```python
from build123d import *

# Parameters (mm, degrees)
F0_W      = 1520
F0_H      = 750
F1_DEPTH  = 25
F2_W      = 1470
F2_H      = 25
F3_DEPTH  = 25
F5_DEPTH  = 65
F7_W      = 25
F7_H      = 25
F8_DEPTH  = 675
F10_DEPTH = 65
F12_W     = 25
F12_H     = 25
F13_DEPTH = 675
F15_W     = 25
F15_H     = 25
F16_DEPTH = 675
F18_W     = 25
F18_H     = 25
F19_DEPTH = 650
F21_W     = 25
F21_H     = 25
F22_DEPTH = 650
F24_DEPTH = 10
F26_DEPTH = 10
F29_DEPTH = 10
F31_DEPTH = 10


with BuildPart() as f1:
    # F0 (on Top) → F1 (new body)
    with BuildSketch(Plane.XY):
        with Locations((-760, 375)):
            Rectangle(F0_W, F0_H)
    extrude(amount=F1_DEPTH)

    # F2 (on face) → F3 (join)
    with BuildSketch(Plane(origin=(0, 0, 0), x_dir=(1, 0, 0), z_dir=(0, 0, -1))):
        with Locations((-760, -37.5)):
            Rectangle(F2_W, F2_H)
        with Locations((-760, -712.5)):
            Rectangle(F2_W, F2_H)
    extrude(amount=F3_DEPTH)

    # F4 (on face) → F5 (join)
    with BuildSketch(Plane(origin=(0, 0, 0), x_dir=(1, 0, 0), z_dir=(0, 0, -1))):
        Polygon((-65, -25), (-25, -25), (-25, -50), (-65, -50), (-65, -52), (-23, -52), (-23, -23), (-65, -23), align=None)
    extrude(amount=F5_DEPTH)

    # F7 (on offset) → F8 (join)
    with BuildSketch(Plane(origin=(0, 0, -35), x_dir=(1, 0, 0), z_dir=(0, 0, -1))):
        with Locations((-37.5, -37.523640207)):
            Rectangle(F7_W, F7_H)
    extrude(amount=F8_DEPTH)

    # F9 (on face) → F10 (join)
    with BuildSketch(Plane.XY):
        Polygon((-1495, 724.9829173088), (-1455, 724.9829173088), (-1455, 726.9829173088), (-1497, 726.9829173088), (-1497, 697.9829173088), (-1455, 697.9829173088), (-1455, 699.9829173088), (-1495, 699.9829173088), align=None)
        Polygon((-65.0490959734, 726.9829173088), (-65.0490959734, 724.9829173088), (-25.0490959734, 724.9829173088), (-25.0490959734, 699.9829173088), (-65.0490959734, 699.9829173088), (-65.0490959734, 697.9829173088), (-23.0490959734, 697.9829173088), (-23.0490959734, 726.9829173088), align=None)
        Polygon((-1455, 25), (-1495, 25), (-1495, 50), (-1455, 50), (-1455, 52), (-1497, 52), (-1497, 23), (-1455, 23), align=None)
    extrude(amount=-F10_DEPTH)

    # F12 (on offset) → F13 (join)
    with BuildSketch(Plane(origin=(0, 0, -35), x_dir=(1, 0, 0), z_dir=(0, 0, -1))):
        with Locations((-1482.5, -37.5)):
            Rectangle(F12_W, F12_H)
    extrude(amount=F13_DEPTH)

    # F15 (on offset) → F16 (join)
    with BuildSketch(Plane(origin=(0, 0, -35), x_dir=(1, 0, 0), z_dir=(0, 0, -1))):
        with Locations((-37.5, -712.5)):
            Rectangle(F15_W, F15_H)
        with Locations((-1482.5, -712.5)):
            Rectangle(F15_W, F15_H)
    extrude(amount=F16_DEPTH)

    # F18 (on offset) → F19 (join)
    with BuildSketch(Plane(origin=(0, 50.023640207, 0), x_dir=(-1, 0, 0), z_dir=(0, 1, 0))):
        with Locations((37.5, -497.5)):
            Rectangle(F18_W, F18_H)
    extrude(amount=F19_DEPTH)

    # F21 (on offset) → F22 (join)
    with BuildSketch(Plane(origin=(0, 50, 0), x_dir=(-1, 0, 0), z_dir=(0, 1, 0))):
        with Locations((1482.5, -497.5)):
            Rectangle(F21_W, F21_H)
    extrude(amount=F22_DEPTH)

    # F23 (on face) → F24 (join)
    with BuildSketch(Plane.XZ.offset(-700)):
        with BuildLine():
            Line((-50, -190.7444713597), (-234.6244849475, -9.2794851613))
            ThreePointArc((-234.6244849475, -9.2794851613), (-246.6039118675, -7.7336055545), (-251.332803081, -18.8481906111))
            Line((-251.332803081, -18.8481906111), (-50, -216.7355636904))
            Line((-50, -216.7355636904), (-50, -190.7444713597))
        make_face()
        with BuildLine():
            Line((-27.8014624786, -212.5631229112), (-50, -190.7444713597))
            Line((-50, -190.7444713597), (-50, -216.7355636904))
            Line((-50, -216.7355636904), (-44.5097806121, -222.131828361))
            ThreePointArc((-44.5097806121, -222.131828361), (-32.5303536921, -223.6777079678), (-27.8014624786, -212.5631229112))
        make_face()
    extrude(amount=F24_DEPTH)

    # F25 (on face) → F26 (join)
    with BuildSketch(Plane(origin=(0, 50.023640207, 0), x_dir=(-1, 0, 0), z_dir=(0, 1, 0))):
        with BuildLine():
            Line((50, -188.6229664357), (50, -216.7160920101))
            Line((50, -216.7160920101), (250.9788283543, -18.4630064225))
            ThreePointArc((250.9788283543, -18.4630064225), (251.07538107, -4.3212004002), (236.9335750477, -4.2246476845))
            Line((236.9335750477, -4.2246476845), (50, -188.6229664357))
        make_face()
        with BuildLine():
            ThreePointArc((30.4773733467, -207.880820631), (30.380820631, -222.0226266533), (44.5226266533, -222.119179369))
            Line((44.5226266533, -222.119179369), (50, -216.7160920101))
            Line((50, -216.7160920101), (50, -188.6229664357))
            Line((50, -188.6229664357), (30.4773733467, -207.880820631))
        make_face()
    extrude(amount=F26_DEPTH)

    # F28 (on offset) → F29 (join)
    with BuildSketch(Plane.XZ.offset(-700)):
        with BuildLine():
            ThreePointArc((-1268.519621658, -19.0091897955), (-1268.3869301053, -4.8676766886), (-1282.5284432121, -4.7349851358))
            Line((-1282.5284432121, -4.7349851358), (-1489.504410777, -207.8628976702))
            ThreePointArc((-1489.504410777, -207.8628976702), (-1489.6371023298, -222.004410777), (-1475.495589223, -222.1371023298))
            Line((-1475.495589223, -222.1371023298), (-1268.519621658, -19.0091897955))
        make_face()
    extrude(amount=F29_DEPTH)

    # F30 (on face) → F31 (join)
    with BuildSketch(Plane(origin=(0, 50, 0), x_dir=(-1, 0, 0), z_dir=(0, 1, 0))):
        with BuildLine():
            ThreePointArc((1475.506314972, -222.1476128693), (1489.6476128693, -221.993685028), (1489.493685028, -207.8523871307))
            Line((1489.493685028, -207.8523871307), (1470, -188.7785095141))
            Line((1470, -188.7785095141), (1470, -216.7598794703))
            Line((1470, -216.7598794703), (1475.506314972, -222.1476128693))
        make_face()
        with BuildLine():
            Line((1470, -216.7598794703), (1470, -188.7785095141))
            Line((1470, -188.7785095141), (1282.212911818, -5.0355213195))
            ThreePointArc((1282.212911818, -5.0355213195), (1268.0716139207, -5.1894491609), (1268.225541762, -19.3307470582))
            Line((1268.225541762, -19.3307470582), (1470, -216.7598794703))
        make_face()
    extrude(amount=F31_DEPTH)


solid = f1.part
```
The model under review builds one solid part; all positions refer to its coordinate system, in mm. A direction names the side the tool comes from. Coordinates: 2 decimals unless noted, no trailing zeros. Write each loop counter-clockwise with the first axis right and the second up, starting at its lowest first coordinate (ties: lowest second). Pieces come first, ordered by that corner, then holes.
1) We need section C-C on x = -382. State the section outline as (y, z) points.
2) To check wall thickness, follow probe 1 along Z at (x, y) = (-784, 348.5). State the ranges of the line that lie inside material, in increasing order.
3) Machinability: for faces 5 (the face through (-141, 700, -113)), 6 (the face through (-54, 724.983, -40)), 7 (the face through (-1497, 38, -32)), 8 (the face through (-23, 38, -32)), which of the approach directions +Z, -Z, +X, -X, +Y, -Y give a long, thin tool a straight path to every point of the face, cutting with its end or side? Answer none if there is none.
4) We need section A-A on z = -588.5. State the section outline as (x, y) points, then the cut area to 3 significant figures.
5) Clearance check with flat-ended pins moving along their axes: pin 1 Ø1.6 at (y, z) = (24, -30) entering from -X; pin 2 Ø12 at (x, y) = (-682.5, 616.5) entering from -Z; pin 3 Ø7.5 at (x, z) = (-33.5, -567.5) entering from +Y. State where each tip first meets the part, or that it passes through.
6) We need section B-B on y = 245. State the section outline as (x, z) points, then the cut area to 4 significant figures.
7) The part is to be moulded in two halves that separate along Y. For faces 1 (the face through (-140, 60.024, -113)), 2 (the face through (-771, 380, 25)), 3 (the face through (-44, 726.983, -32)), 4 (the face through (-1479.2, 699.7, -65)), say which applies: pulls with the +Y half, pulls with the -Y half, needs draft (parallel to the pull), parting line crosses it, or undercut.
Answer list:
1. outline: (0, 0) - (25, 0) - (25, -25) - (50, -25) - (50, 0) - (700, 0) - (700, -25) - (725, -25) - (725, 0) - (750, 0) - (750, 25) - (0, 25) - close
2. probe 1: z = 0 to 25
3. face 5: -Z, +Y
3. face 6: none
3. face 7: -Z, -X, +Y, -Y
3. face 8: -Z, +X, +Y, -Y
4. outline: (-1495, 25) - (-1470, 25) - (-1470, 50) - (-1495, 50) - close; (-1495, 700) - (-1470, 700) - (-1470, 725) - (-1495, 725) - close; (-50, 25.02) - (-25, 25.02) - (-25, 50.02) - (-50, 50.02) - close; (-50, 700) - (-25, 700) - (-25, 725) - (-50, 725) - close
4. area: 2,500 mm2
5. pin 1: stops at x = -1497
5. pin 2: stops at z = 0
5. pin 3: stops at y = 725
6. outline: (-1520, 0) - (0, 0) - (0, 25) - (-1520, 25) - close; (-1495, -510) - (-1470, -510) - (-1470, -485) - (-1495, -485) - close; (-50, -510) - (-25, -510) - (-25, -485) - (-50, -485) - close
6. area: 39,250 mm2
7. face 1: undercut
7. face 2: needs draft
7. face 3: pulls with the +Y half
7. face 4: undercut
